Could you check a few things on this model? Use its own coordinates, in mm. Face numbers are marked on the shaded views. A direction names the side the tool comes from. Give positions to 0.01 mm unless a question says otherwise; leave off trailing zeros. Loops run counter-clockwise (first coordinate to the right, second up) from the corner with the lowest first, then second, coordinate; pieces in that order, holes last. Notation, with made-up numbers: M 70,76.5 L 91,76.5 A17 ccw 91,103.5 Z; hole C 15.25,28.5 d11. An arc over 180 degrees is marked long. Answer in a Markdown table with one row per item. Add a question column.
```python
from build123d import *

# Parameters (mm, degrees)
SKETCH1_W                        = 127
SKETCH1_H                        = 152.4
BOSS_EXTRUDE1_DEPTH              = 12.7
SKETCH2_R                        = 7.9375
CUT_EXTRUDE1_DEPTH               = 166.587741092
SKETCH3_W                        = 127
SKETCH3_H                        = 3.175
BOSS_EXTRUDE2_DEPTH              = 12.7
SKETCH4_W                        = 38.1
SKETCH4_H                        = 12.7
CUT_EXTRUDE2_DEPTH               = 107.172778556
FILLET1_R                        = 6.35
F_1_4_20_TAPPED_HOLE1_AT_2_COUNT = 2
F_1_4_20_TAPPED_HOLE1_AT_2_PITCH = 38.1
SKETCH7_W                        = 12.7
SKETCH7_H                        = 19.05
BOSS_EXTRUDE3_DEPTH              = 12.7
SKETCH8_R                        = 0.79375
CUT_EXTRUDE3_DEPTH               = 115.222803793


with BuildPart() as part:
    # Sketch1 → Boss-Extrude1 (new body)
    with BuildSketch(Plane.XY):
        with Locations((0, 76.2)):
            Rectangle(SKETCH1_W, SKETCH1_H)
    extrude(amount=BOSS_EXTRUDE1_DEPTH)

    # Sketch2 → Cut-Extrude1 (cut, through all)
    with BuildSketch(Plane.XY.offset(12.7)):
        with BuildLine():
            Line((-63.5, 152.4), (-63.5, 56.977000238))
            Line((-63.5, 56.977000238), (-17.807704814, 79.918060357))
            ThreePointArc((-17.807704814, 79.918060357), (0, 84.1375), (17.807704814, 79.918060357))
            Line((17.807704814, 79.918060357), (63.5, 56.977000238))
            Line((63.5, 56.977000238), (63.5, 152.4))
            Line((63.5, 152.4), (-63.5, 152.4))
        make_face()
        with Locations((0, 44.45)):
            Circle(SKETCH2_R)
    extrude(amount=-CUT_EXTRUDE1_DEPTH, mode=Mode.SUBTRACT)

    # Sketch3 → Boss-Extrude2 (add)
    with BuildSketch(Plane(origin=(0, 0, 0), x_dir=(-1, 0, 0), z_dir=(0, 0, -1))):
        with Locations((0, -1.5875)):
            Rectangle(SKETCH3_W, SKETCH3_H)
    extrude(amount=-BOSS_EXTRUDE2_DEPTH)

    # Sketch4 → Cut-Extrude2 (cut, through all)
    with BuildSketch(Plane.XY.offset(12.7)):
        with Locations((0, 3.175)):
            Rectangle(SKETCH4_W, SKETCH4_H)
    extrude(amount=-CUT_EXTRUDE2_DEPTH, mode=Mode.SUBTRACT)

    # Fillet1
    fillet1_edges = [part.edges().sort_by_distance(p)[0] for p in [
        (-19.05, 9.525, 6.35),
        (19.05, 9.525, 6.35),
    ]]
    fillet(fillet1_edges, radius=FILLET1_R)
    fillet1_2_edges = [part.edges().sort_by_distance(p)[0] for p in [
        (-19.05, -3.175, 6.35),
        (19.05, -3.175, 6.35),
    ]]
    fillet(fillet1_2_edges, radius=FILLET1_R - 0.0001)  # a hair under: the kernel refuses the full size

    # Sketch5 → 1/4-20 Tapped Hole1 (revolve, cut)
    with BuildSketch(Plane(origin=(63.5, 45.951000119, 6.35), x_dir=(0, 0, -1), z_dir=(0, 1, 0))):
        Polygon((0, 0), (0, 18.043816902), (2.5527, 16.51), (2.5527, 0), align=None)
    f_1_4_20_tapped_hole1 = revolve(axis=Axis((69.85, 45.951000119, 6.35), (-1, 0, 0)), mode=Mode.SUBTRACT)

    # 1/4-20 Tapped Hole1 at 2: 1/4-20 Tapped Hole1 ×2
    with Locations(*[(0, -i * F_1_4_20_TAPPED_HOLE1_AT_2_PITCH, 0) for i in range(1, F_1_4_20_TAPPED_HOLE1_AT_2_COUNT)]):
        add(f_1_4_20_tapped_hole1, mode=Mode.SUBTRACT)

    # Sketch7 → Boss-Extrude3 (add)
    with BuildSketch(Plane(origin=(63.5, 0, 0), x_dir=(0, 0, -1), z_dir=(1, 0, 0))):
        with Locations((-6.35, 26.901000119)):
            Rectangle(SKETCH7_W, SKETCH7_H)
    boss_extrude3 = extrude(amount=BOSS_EXTRUDE3_DEPTH)

    # Sketch8 → Cut-Extrude3 (cut, through all)
    with BuildSketch(Plane.XY.offset(12.7)):
        with Locations((63.5, 37.219750119)):
            Circle(SKETCH8_R)
        with Locations((63.5, 16.582250119)):
            Circle(SKETCH8_R)
    cut_extrude3 = extrude(amount=-CUT_EXTRUDE3_DEPTH, mode=Mode.SUBTRACT)

    # Mirror1: 1/4-20 Tapped Hole1, Boss-Extrude3, Cut-Extrude3 across plane
    add(f_1_4_20_tapped_hole1.mirror(Plane(origin=(0, 0, 0), x_dir=(0, 0, 1), z_dir=(1, 0, 0))), mode=Mode.SUBTRACT)
    add(boss_extrude3.mirror(Plane(origin=(0, 0, 0), x_dir=(0, 0, 1), z_dir=(1, 0, 0))))
    add(cut_extrude3.mirror(Plane(origin=(0, 0, 0), x_dir=(0, 0, 1), z_dir=(1, 0, 0))), mode=Mode.SUBTRACT)

    # Mirror1 copy 1 sketch → Mirror1 copy 1 (revolve, cut)
    with BuildSketch(Plane(origin=(-63.5, 7.851000119, 6.35), x_dir=(0, 0, -1), z_dir=(0, 1, 0))):
        Polygon((0, 0), (0, -18.043816902), (2.5527, -16.51), (2.5527, 0), align=None)
    revolve(axis=Axis((-69.85, 7.851000119, 6.35), (-1, 0, 0)), mode=Mode.SUBTRACT)


solid = part.part
```
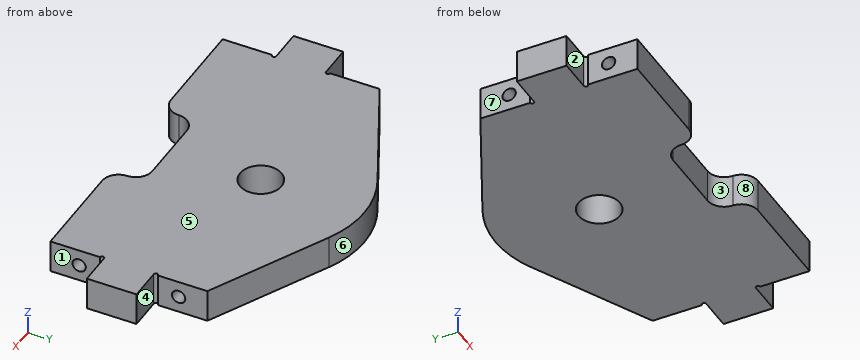
Item 1: Suppose I cut it at B-B (x = 58.5). List the corners of the cut face in (y, z) for me (3 decimals).
Item 2: For P1, Ø12, axis at x = -52, y = 71, coming from the -Z side; P2, Ø6, axis at y = 7.851, z = 6.35, coming from the +X side; P3, Ø3, axis at y = 45.951, z = 6.35, coming from the -X side; P4, Ø4, axis at y = 5, z = 3.5, coming from the -X side, each with a flat end and sliding along its axis, tell me the tip position at first contact or that it passes through.
Item 3: For the marked faces 1, 2, 3 and 4, which set-ups out of +Z, -Z, +X, -X, +Y, -Y let a thin tool reach every point of the face, with its end or its side?
Item 4: Suppose I cut it at A-A (x = 0). List the corners of the cut face in (y, z) for me (1 decimal), then the cut area to 3 significant figures.
Item 5: Suppose I cut it at D-D (x = -23). List the corners of the cut face in (y, z) for me.
Item 6: If we mould it in two halves opening along X, with no side actions, what happens to the marked faces 5, 6, 7 and 8? For each: +X half, -X half, draft (parallel to the pull), parting line (faces both ways), or undercut.
Item 7: I need wall thicknesses on L1, parallel to Y at x = 59.75, z = 6.35 (3 decimals); L2, parallel to Y at x = 0, z = 6.75 (1 decimal); L3, parallel to Y at x = 51.25, z = 6.35 (3 decimals). Which ranges of each line are inside material? Lowest first, please.
Item 8: Suppose I cut it at C-C (y = 76). List the corners of the cut face in (x, z) for me.
Values found:
| question | item | result |
|---|---|---|
| 1 | outline | M -3.175,0 L 59.487,0 L 59.487,12.7 L -3.175,12.7 Z; hole C 7.851,6.35 d5.105; hole C 45.951,6.35 d5.105 |
| 2 | P1 | through |
| 2 | P2 | x = 63.5 |
| 2 | P3 | x = -46.36 |
| 2 | P4 | x = -63.5 |
| 3 | face 1 | +Z, -Z, +X, -Y |
| 3 | face 2 | +Z, -Z, -X, -Y |
| 3 | face 3 | +Z, -Z, -Y |
| 3 | face 4 | +Z, -Z, +X, +Y |
| 4 | outline | M 9.5,0 L 36.5,0 L 36.5,12.7 L 9.5,12.7 Z; M 52.4,0 L 84.1,0 L 84.1,12.7 L 52.4,12.7 Z |
| 4 | area | 746 mm² |
| 5 | outline | M -2.7,0 L 77.31,0 L 77.31,12.7 L -2.7,12.7 Z |
| 6 | face 5 | draft |
| 6 | face 6 | parting line |
| 6 | face 7 | -X half |
| 6 | face 8 | undercut |
| 7 | L1 | -3.175 to 5.298, 10.404 to 43.398, 48.504 to 58.86 |
| 7 | L2 | 9.5 to 36.5, 52.4 to 84.1 |
| 7 | L3 | -3.175 to 5.298, 10.404 to 43.398, 48.504 to 63.127 |
| 8 | outline | M -25.61,0 L 25.61,0 L 25.61,12.7 L -25.61,12.7 Z |
